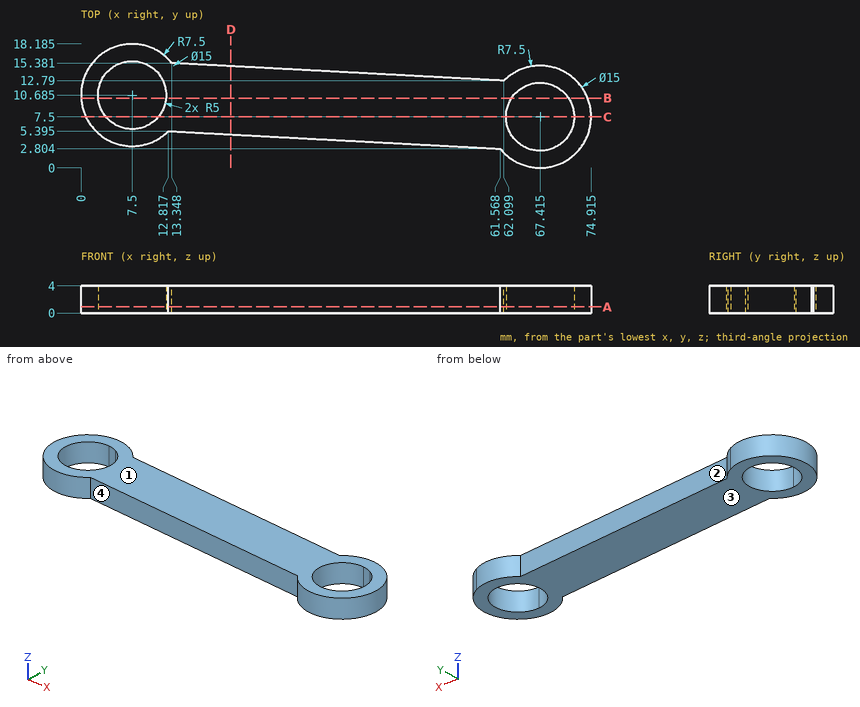
Could you check a few things on this drawing? It's one solid part, dimensions in mm from its lowest x, y, z. A direction names the side the tool comes from. Give positions to 0.01 mm unless a question says otherwise; leave off trailing zeros. Loops run counter-clockwise (first coordinate to the right, second up) from the corner with the lowest first, then second, coordinate; pieces in that order, holes last. Notation, with made-up numbers: M 80.25,-36 L 84.25,-36 A24 cw 84.25,-17 Z; hole C 75,81.25 d10. An arc over 180 degrees is marked long. Answer as a JSON object with one key per item and string values.
Q1. For the marked faces 1 and 2, which set-ups out of +Z, -Z, +X, -X, +Y, -Y let a thin tool reach every point of the face, with its end or its side?
Values found:
{"face 1": "+Z, +X, -X, +Y, -Y", "face 2": "+Z, -Z, +Y"}
Q2. Suppose I cut it at D-D, the plane x = 22. List the corners of the cut face in (y, z) for me.
Values found:
{"outline": "M 4.91,0 L 14.92,0 L 14.92,4 L 4.91,4 Z"}
Q3. Suppose I cut it at B-B, the plane y = 10.25. List the corners of the cut face in (x, z) for me, plus the area to 3 significant figures.
Values found:
{"outline": "M 0.01,0 L 2.52,0 L 2.52,4 L 0.01,4 Z; M 12.48,0 L 63.24,0 L 63.24,4 L 12.48,4 Z; M 71.59,0 L 74.39,0 L 74.39,4 L 71.59,4 Z", "area": "224 mm²"}
Q4. If I drill on probe 1 along X at (y, z) = (10, 1.95) (1 decimal); probe 2 along X at (y, z) = (8, 1.3) (1 decimal); probe 3 along Y at (x, z) = (68, 1) (1 decimal), over which ranges is the centre line in solid material (lowest first)? Write a range as [from, to].
Values found:
{"probe 1": "x = [0, 2.5], [12.5, 63.1], [71.7, 74.5]", "probe 2": "x = [0.5, 3.3], [11.7, 62.4], [72.4, 74.9]", "probe 3": "y = [0, 2.5], [12.5, 15]"}
Q5. If we mould it in two halves opening along X, with no side actions, what happens to the marked faces 3 and 4? For each: pulls with the +X half, pulls with the -X half, needs draft (parallel to the pull), parting line crosses it, or undercut.
Values found:
{"face 3": "needs draft", "face 4": "undercut"}
Q6. For P1, Ø1, axis at x = 51, z = 0.5, coming from the +Y side; P2, Ø1, axis at y = 14, z = 3, coming from the -X side, each with a flat end and sliding along its axis, tell me the tip position at first contact or that it passes through.
Values found:
{"P1": "stops at y = 13.41", "P2": "stops at x = 0.55"}
Q7. Suppose I cut it at A-A, the plane z = 0.9. State how many separate pieces and enclosed holes the cut face has.
Values found:
{"separate pieces": "1", "enclosed holes": "2"}
Q8. Suppose I cut it at C-C, the plane y = 7.5. List the corners of the cut face in (x, z) for me (1 decimal), plus the area to 3 significant figures.
Values found:
{"outline": "M 0.7,0 L 3.6,0 L 3.6,4 L 0.7,4 Z; M 11.4,0 L 62.4,0 L 62.4,4 L 11.4,4 Z; M 72.4,0 L 74.9,0 L 74.9,4 L 72.4,4 Z", "area": "226 mm²"}
